```python
from build123d import *

# Parameters (mm, degrees)
F0_W      = 895.35
F0_H      = 958.85
F1_DEPTH  = 12.7
F2_W      = 257.048
F2_H      = 76.2
F2_R      = 8.73125
F3_DEPTH  = 57.15
F6_DEPTH  = 12.7
F8_DEPTH  = 12.7
F9_W      = 19.05
F9_H      = 552.45
F10_DEPTH = 946.278
F13_DEPTH = 19.05
F14_W     = 69.85
F14_H     = 800.1
F14_W_2   = 95.25
F15_DEPTH = 25.4


with BuildPart() as f1:
    # F0 (on Top) → F1 (new body)
    with BuildSketch(Plane.XY):
        Rectangle(F0_W, F0_H)
    extrude(amount=F1_DEPTH)

    # F2 (on face) → F3 (join)
    with BuildSketch(Plane.XY.offset(12.7)):
        with Locations((307.975, -146.05)):
            Rectangle(F2_W, F2_H)
        with Locations((205.613, -146.812)):
            Circle(F2_R, mode=Mode.SUBTRACT)
        with Locations((410.337, -146.812)):
            Circle(F2_R, mode=Mode.SUBTRACT)
        with Locations((307.975, -317.5)):
            Rectangle(F2_W, F2_H)
        with Locations((205.613, -316.738)):
            Circle(F2_R, mode=Mode.SUBTRACT)
        with Locations((410.337, -316.738)):
            Circle(F2_R, mode=Mode.SUBTRACT)
        with Locations((307.975, 146.05)):
            Rectangle(F2_W, F2_H)
        with Locations((205.613, 146.812)):
            Circle(F2_R, mode=Mode.SUBTRACT)
        with Locations((410.337, 146.812)):
            Circle(F2_R, mode=Mode.SUBTRACT)
        with Locations((307.975, 317.5)):
            Rectangle(F2_W, F2_H)
        with Locations((205.613, 316.738)):
            Circle(F2_R, mode=Mode.SUBTRACT)
        with Locations((410.337, 316.738)):
            Circle(F2_R, mode=Mode.SUBTRACT)
    extrude(amount=F3_DEPTH)

    # F5 (on offset) → F6 (join)
    with BuildSketch(Plane.XZ.offset(454.152)):
        Polygon((-447.675, 247.65), (-447.675, 12.7), (436.499, 12.7), (436.499, 38.1), (-371.475, 247.65), align=None)
    extrude(amount=F6_DEPTH)

    # F7 (on face) → F8 (join)
    with BuildSketch(Plane.XZ.offset(466.852)):
        Polygon((436.499, -76.2), (436.499, 0), (-447.675, 0), (-447.675, -552.45), (-371.475, -552.45), align=None)
    extrude(amount=-F8_DEPTH)

    # F9 (on face) → F10 (cut, through all)
    with BuildSketch(Plane.XZ.offset(466.852)):
        with Locations((-438.15, -276.225)):
            Rectangle(F9_W, F9_H)
    extrude(amount=-F10_DEPTH, mode=Mode.SUBTRACT)

    # F11: F1 across plane


with BuildPart() as f1_1:
    add(f1.part)
    add(f1.part.mirror(Plane.XZ))

    # F12 (on face) → F13 (join)
    with BuildSketch(Plane(origin=(-428.625, 0, 0), x_dir=(0, -1, 0), z_dir=(-1, 0, 0))):
        with BuildLine():
            Line((479.425, -552.45), (479.425, 0))
            Line((479.425, 0), (-479.425, 0))
            Line((-479.425, 0), (-479.425, -552.45))
            Line((-479.425, -552.45), (-365.125, -552.45))
            Line((-365.125, -552.45), (-365.125, -241.3))
            ThreePointArc((-365.125, -241.3), (-350.2460244843, -205.3789755157), (-314.325, -190.5))
            Line((-314.325, -190.5), (314.325, -190.5))
            ThreePointArc((314.325, -190.5), (350.2460244843, -205.3789755157), (365.125, -241.3))
            Line((365.125, -241.3), (365.125, -552.45))
            Line((365.125, -552.45), (479.425, -552.45))
        make_face()
    extrude(amount=F13_DEPTH)

    # F14 (on face) → F15 (join)
    with BuildSketch(Plane(origin=(-447.675, 0, 0), x_dir=(0, -1, 0), z_dir=(-1, 0, 0))):
        with Locations((431.927, -152.4)):
            Rectangle(F14_W, F14_H)
        with Locations((-419.227, -152.4)):
            Rectangle(F14_W_2, F14_H)
    extrude(amount=F15_DEPTH)


solid = f1_1.part
```
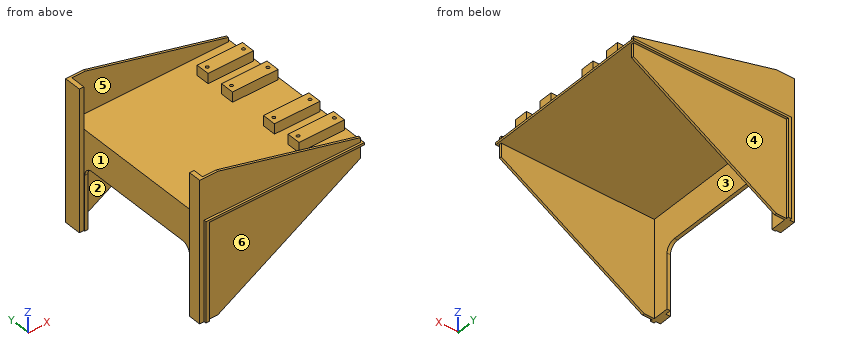
Geometry: final body of the model. Coordinates: model frame, mm. Face numbers are marked on the shaded views. A direction names the side the tool comes from. Round coordinates to 2 decimals unless told otherwise and drop trailing zeros. Order: outer loops, then holes, each group sorted by start corner. A loop starts at its lowest first (then second) coordinate and runs counter-clockwise, first axis right, second up. Notation, with made-up numbers: (84, -21) -> (114, -21) arc R29 ccw to (114, 4) -> close; hole circle Ø3 at (40, 63). An arc over 180 degrees is marked (long way). Write each question's results on one line, items separated by ' | '.
Q1. Access query for the marked faces 1 and 2. Directions: +Z, -Z, +X, -X, +Y, -Y. A direction counts if a zero-diameter tool reaches every point of the face in a straight line with its end or side. Return the directions, or none.
Response values:
face 1: +Z, -Z, -X | face 2: -Z, +X
Q2. Section query B-B (y = 393.5). Output: boundary loops of the cut face in (x, z) (3 decimals).
Response values:
outline: (-473.075, -552.45) -> (-428.625, -552.45) -> (-428.625, 0) -> (447.675, 0) -> (447.675, 12.7) -> (-447.675, 12.7) -> (-447.675, 247.65) -> (-473.075, 247.65) -> close
Q3. Section query A-A (z = 196.5). Output: boundary loops of the cut face in (x, y) (3 decimals), and give its area (3 significant figures).
Response values:
outline: (-473.075, -466.852) -> (-174.253, -466.852) -> (-174.253, -454.152) -> (-447.675, -454.152) -> (-447.675, -397.002) -> (-473.075, -397.002) -> close; (-473.075, 371.602) -> (-447.675, 371.602) -> (-447.675, 454.152) -> (-174.253, 454.152) -> (-174.253, 466.852) -> (-473.075, 466.852) -> close | area: 11,100 mm²
Q4. Ray query, line 1 along Y through (x, z) = (-236, -412.5); line 2 along Z through (x, y) = (149, -165.5); line 3 along X through (y, z) = (156, -74) (3 decimals). Return the intervals inside material, ascending.
Response values:
line 1: -466.85 to -454.15, 454.15 to 466.85 | line 2: 0 to 12.7 | line 3: -447.675 to -428.625
Q5. Pull-direction query (Y, two-part tool) for the marked faces 3, 4, 5 and 6; classes: released by +Y, released by -Y, zero draft, split by the parting line, or undercut.
Response values:
face 3: undercut | face 4: released by +Y | face 5: undercut | face 6: released by -Y
Q6. Section query D-D (x = -85.5). Output: boundary loops of the cut face in (y, z) (3 decimals), and give its area (3 significant figures).
Response values:
outline: (-479.425, 0) -> (-466.852, 0) -> (-466.852, -383.886) -> (-454.152, -383.886) -> (-454.152, 0) -> (454.152, 0) -> (454.152, -383.886) -> (466.852, -383.886) -> (466.852, 0) -> (479.425, 0) -> (479.425, 12.7) -> (466.852, 12.7) -> (466.852, 173.482) -> (454.152, 173.482) -> (454.152, 12.7) -> (-454.152, 12.7) -> (-454.152, 173.482) -> (-466.852, 173.482) -> (-466.852, 12.7) -> (-479.425, 12.7) -> close | area: 26,000 mm²
Q7. Section query C-C (z = -147.5). Output: boundary loops of the cut face in (x, y) (3 decimals).
Response values:
outline: (-473.075, -466.852) -> (-447.675, -466.852) -> (-447.675, -479.425) -> (-428.625, -479.425) -> (-428.625, -466.852) -> (315.536, -466.852) -> (315.536, -454.152) -> (-428.625, -454.152) -> (-428.625, 454.152) -> (315.536, 454.152) -> (315.536, 466.852) -> (-428.625, 466.852) -> (-428.625, 479.425) -> (-447.675, 479.425) -> (-447.675, 466.852) -> (-473.075, 466.852) -> (-473.075, 371.602) -> (-447.675, 371.602) -> (-447.675, -397.002) -> (-473.075, -397.002) -> close
Q8. Pin query (flat end, axial travel): pin 1 Ø22.5 at (x, y) = (410.337, 316.738) entering from -Z; pin 2 Ø5 at (x, z) = (-287, -300) entering from -Y; pin 3 Ø10 at (x, y) = (37, 275.5) entering from +Z. Return the tip coordinate at first contact, or that it passes through.
Response values:
pin 1: z = 0 | pin 2: y = -466.85 | pin 3: z = 12.7
